```python
from build123d import *

# Parameters (mm, degrees)
EXTRUDE_1_DEPTH        = 60
HOLE_WIZARD_M3_1_D     = 2.5
HOLE_WIZARD_M3_1_DEPTH = 15
HOLE_WIZARD_M3_1_TIP   = 0.751075774
HOLE_WIZARD_M3_2_D     = 2.5
HOLE_WIZARD_M3_2_DEPTH = 15
HOLE_WIZARD_M3_2_TIP   = 0.751075774


with BuildPart() as part:
    # 草图1 → 凸台-拉伸1 (new body)
    with BuildSketch(Plane.XY):
        Polygon((1.363201019, 2.23742776), (-1.25606877, 2.299280593), (-2.619269789, 0.061852833), (-1.363201019, -2.23742776), (1.25606877, -2.299280593), (2.619269789, -0.061852833), align=None)
    extrude(amount=EXTRUDE_1_DEPTH)

    # M3 螺纹孔1
    with Locations(Plane.XY.offset(60)):
        with Locations((0, 0)):
            Hole(HOLE_WIZARD_M3_1_D / 2, depth=HOLE_WIZARD_M3_1_DEPTH)
            with Locations((0, 0, -(HOLE_WIZARD_M3_1_DEPTH + HOLE_WIZARD_M3_1_TIP / 2))):  # 118° drill point
                Cone(0, HOLE_WIZARD_M3_1_D / 2, HOLE_WIZARD_M3_1_TIP, mode=Mode.SUBTRACT)

    # M3 螺纹孔2
    with Locations(Plane(origin=(0, 0, 0), x_dir=(-1, 0, 0), z_dir=(0, 0, -1))):
        with Locations((0, 0)):
            Hole(HOLE_WIZARD_M3_2_D / 2, depth=HOLE_WIZARD_M3_2_DEPTH)
            with Locations((0, 0, -(HOLE_WIZARD_M3_2_DEPTH + HOLE_WIZARD_M3_2_TIP / 2))):  # 118° drill point
                Cone(0, HOLE_WIZARD_M3_2_D / 2, HOLE_WIZARD_M3_2_TIP, mode=Mode.SUBTRACT)


solid = part.part
```
Geometry check sheet. Reference: the model listing, model coordinates, mm. A direction names the side the tool comes from. Coordinates: 2 decimals unless noted, no trailing zeros. Order: outer loops, then holes, each group sorted by start corner. A loop starts at its lowest first (then second) coordinate and runs counter-clockwise, first axis right, second up.
Q1. Tool access check on faces 4 (the face through (-0.27, -1.22, 7.6)), 5 (the face through (1.928, -1.196, 29.58)), 6 (the face through (0.27, -1.22, 52.4)). Record the directions out of +Z, -Z, +X, -X, +Y, -Y that give a thin tool (end or side, any length) a straight path to the whole face; none if there is none.
Reply:
face 4: -Z
face 5: +Z, -Z, +X, -Y
face 6: +Z
Q2. Sectioned sample at C-C on y = 1.75. Record the cut outline in (x, z), and give its area (3 significant figures).
Reply:
outline: (-1.59, 0) - (1.63, 0) - (1.63, 60) - (-1.59, 60) - close
area: 193 mm2
Q3. Sectioned sample at B-B on z = 21. Record the cut outline in (x, y).
Reply:
outline: (-2.62, 0.06) - (-1.36, -2.24) - (1.26, -2.3) - (2.62, -0.06) - (1.36, 2.24) - (-1.26, 2.3) - close
Q4. Draft check along X on faces 1 (the face through (2, 1.07, 29.58)), 2 (the face through (-0.05, -0.21, 44.38)), 3 (the face through (1, 1, 0)). Enter one of: released by +X, released by -X, zero draft, split by the parting line, or undercut.
Reply:
face 1: released by +X
face 2: undercut
face 3: zero draft
Q5. Depth check by flat-ended pin: pin 1 Ø2 at (x, z) = (0, 46) entering from +Y; pin 2 Ø1.5 at (x, y) = (0, 0) entering from +Z; pin 3 Ø2 at (x, y) = (0, 0) entering from +Z. Enter the tip coordinate at first touch or a pass-through.
Reply:
pin 1: stops at y = 2.29
pin 2: stops at z = 44.7
pin 3: stops at z = 44.85
Q6. Sectioned sample at A-A on z = 4.5. Record the cut outline in (x, y).
Reply:
outline: (-2.62, 0.06) - (-1.36, -2.24) - (1.26, -2.3) - (2.62, -0.06) - (1.36, 2.24) - (-1.26, 2.3) - close; hole circle Ø2.5 at (0, 0)
Q7. Thickness scan on probe 1 along X at (y, z) = (-0.1, 54.5); probe 2 along Y at (x, z) = (-1.15, 28.5); probe 3 along X at (y, z) = (0, 56). Record the ranges inside material, lowest first.
Reply:
probe 1: x = -2.53 to -1.25, 1.25 to 2.6
probe 2: y = -2.24 to 2.3
probe 3: x = -2.59 to -1.25, 1.25 to 2.59
